```python
from build123d import *

# Parameters (mm, degrees)
F2_W     = 60.64
F2_H     = 2.8
F2_W_2   = 2.8
F2_H_2   = 60.64
F2_W_3   = 7.58
F2_H_3   = 7.58
F3_DEPTH = 2.8
F4_DEPTH = 6
F5_DEPTH = 35.6
F7_W     = 60.64
F7_H     = 2.8
F7_W_2   = 2.8
F7_H_2   = 60.64
F7_H_3   = 7.58
F7_W_3   = 7.58
F8_DEPTH = 2.8
F9_DEPTH = 6


with BuildPart() as f3:
    # F2 (on Top) → F3 (new body)
    with BuildSketch(Plane.XY):
        with Locations((0, 39.3)):
            Rectangle(F2_W, F2_H)
        Polygon((-40.7, 30.32), (-37.9, 30.32), (-37.9, 37.9), (-30.32, 37.9), (-30.32, 40.7), (-40.7, 40.7), align=None)
        Polygon((37.9, 37.9), (37.9, 30.32), (40.7, 30.32), (40.7, 40.7), (30.32, 40.7), (30.32, 37.9), align=None)
        with Locations((39.3, 0)):
            Rectangle(F2_W_2, F2_H_2)
        Polygon((37.9, -30.32), (37.9, -37.9), (30.32, -37.9), (30.32, -40.7), (40.7, -40.7), (40.7, -30.32), align=None)
        with Locations((0, -39.3)):
            Rectangle(F2_W, F2_H)
        Polygon((-30.32, -40.7), (-30.32, -37.9), (-37.9, -37.9), (-37.9, -30.32), (-40.7, -30.32), (-40.7, -40.7), align=None)
        with Locations((-39.3, 0)):
            Rectangle(F2_W_2, F2_H_2)
        with Locations((34.11, -34.11)):
            Rectangle(F2_W_3, F2_H_3)
        with Locations((34.11, 34.11)):
            Rectangle(F2_W_3, F2_H_3)
        with Locations((-34.11, 34.11)):
            Rectangle(F2_W_3, F2_H_3)
        with Locations((-34.11, 0)):
            Rectangle(F2_W_3, F2_H_2)
        with Locations((34.11, 0)):
            Rectangle(F2_W_3, F2_H_2)
        with Locations((-34.11, -34.11)):
            Rectangle(F2_W_3, F2_H_3)
        with Locations((0, -34.11)):
            Rectangle(F2_W, F2_H_3)
        with Locations((0, 34.11)):
            Rectangle(F2_W, F2_H_3)
    extrude(amount=F3_DEPTH)

    # F2 (on Top) → F4 (join)
    with BuildSketch(Plane.XY):
        with Locations((0, 39.3)):
            Rectangle(F2_W, F2_H)
        Polygon((-40.7, 30.32), (-37.9, 30.32), (-37.9, 37.9), (-30.32, 37.9), (-30.32, 40.7), (-40.7, 40.7), align=None)
        with Locations((-39.3, 0)):
            Rectangle(F2_W_2, F2_H_2)
        Polygon((-30.32, -40.7), (-30.32, -37.9), (-37.9, -37.9), (-37.9, -30.32), (-40.7, -30.32), (-40.7, -40.7), align=None)
        with Locations((0, -39.3)):
            Rectangle(F2_W, F2_H)
        Polygon((37.9, -30.32), (37.9, -37.9), (30.32, -37.9), (30.32, -40.7), (40.7, -40.7), (40.7, -30.32), align=None)
        with Locations((39.3, 0)):
            Rectangle(F2_W_2, F2_H_2)
        Polygon((37.9, 37.9), (37.9, 30.32), (40.7, 30.32), (40.7, 40.7), (30.32, 40.7), (30.32, 37.9), align=None)
    extrude(amount=F4_DEPTH)

    # F2 (on Top) → F5 (join)
    with BuildSketch(Plane.XY):
        Polygon((-40.7, 30.32), (-37.9, 30.32), (-37.9, 37.9), (-30.32, 37.9), (-30.32, 40.7), (-40.7, 40.7), align=None)
        Polygon((37.9, 37.9), (37.9, 30.32), (40.7, 30.32), (40.7, 40.7), (30.32, 40.7), (30.32, 37.9), align=None)
        Polygon((37.9, -30.32), (37.9, -37.9), (30.32, -37.9), (30.32, -40.7), (40.7, -40.7), (40.7, -30.32), align=None)
        Polygon((-30.32, -40.7), (-30.32, -37.9), (-37.9, -37.9), (-37.9, -30.32), (-40.7, -30.32), (-40.7, -40.7), align=None)
    extrude(amount=F5_DEPTH)

    # F7 (on offset) → F8 (join)
    with BuildSketch(Plane.XY.offset(35.6)):
        Polygon((37.9, -30.32), (37.9, -37.9), (30.32, -37.9), (30.32, -40.7), (40.7, -40.7), (40.7, -30.32), align=None)
        with Locations((0, -39.3)):
            Rectangle(F7_W, F7_H)
        with Locations((39.3, 0)):
            Rectangle(F7_W_2, F7_H_2)
        Polygon((-30.32, -40.7), (-30.32, -37.9), (-37.9, -37.9), (-37.9, -30.32), (-40.7, -30.32), (-40.7, -40.7), align=None)
        Polygon((37.9, 37.9), (37.9, 30.32), (40.7, 30.32), (40.7, 40.7), (30.32, 40.7), (30.32, 37.9), align=None)
        with Locations((-39.3, 0)):
            Rectangle(F7_W_2, F7_H_2)
        with Locations((0, 39.3)):
            Rectangle(F7_W, F7_H)
        Polygon((-40.7, 30.32), (-37.9, 30.32), (-37.9, 37.9), (-30.32, 37.9), (-30.32, 40.7), (-40.7, 40.7), align=None)
        with Locations((0, 34.11)):
            Rectangle(F7_W, F7_H_3)
        with Locations((34.11, 34.11)):
            Rectangle(F7_W_3, F7_H_3)
        with Locations((34.11, 0)):
            Rectangle(F7_W_3, F7_H_2)
        with Locations((34.11, -34.11)):
            Rectangle(F7_W_3, F7_H_3)
        with Locations((0, -34.11)):
            Rectangle(F7_W, F7_H_3)
        with Locations((-34.11, -34.11)):
            Rectangle(F7_W_3, F7_H_3)
        with Locations((-34.11, 0)):
            Rectangle(F7_W_3, F7_H_2)
        with Locations((-34.11, 34.11)):
            Rectangle(F7_W_3, F7_H_3)
    extrude(amount=-F8_DEPTH)

    # F7 (on offset) → F9 (join)
    with BuildSketch(Plane.XY.offset(35.6)):
        Polygon((-30.32, -40.7), (-30.32, -37.9), (-37.9, -37.9), (-37.9, -30.32), (-40.7, -30.32), (-40.7, -40.7), align=None)
        with Locations((-39.3, 0)):
            Rectangle(F7_W_2, F7_H_2)
        with Locations((0, -39.3)):
            Rectangle(F7_W, F7_H)
        with Locations((39.3, 0)):
            Rectangle(F7_W_2, F7_H_2)
        with Locations((0, 39.3)):
            Rectangle(F7_W, F7_H)
    extrude(amount=-F9_DEPTH)


solid = f3.part
```
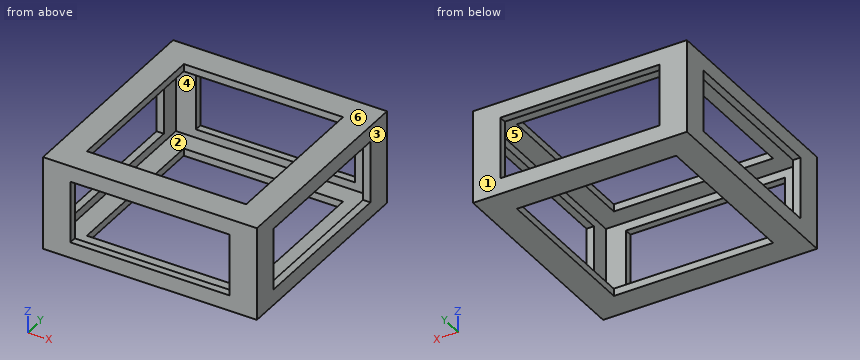
Geometry check sheet. Reference: the model listing, model coordinates, mm. Face numbers are marked on the shaded views. A direction names the side the tool comes from. Coordinates: 2 decimals unless noted, no trailing zeros. Write each loop counter-clockwise with the first axis right and the second up, starting at its lowest first coordinate (ties: lowest second). Pieces come first, ordered by that corner, then holes. Notation, with made-up numbers: M 45,-33.5 L 68,-33.5 A7 ccw 68,-22.5 Z; hole C 38,62.25 d5. An arc over 180 degrees is marked long. One line per item, written item: value. Start each with the question number.
(1) Sectioned sample at B-B, the plane x = -7. Enter the section's corners in (y, z), and give its area (3 significant figures).
(2) Release check for a two-part mould opening along Z. For the marked faces 3, 4, 5 and 6 record: released by +Z, released by -Z, zero draft, split by the parting line, or undercut.
(3) Sectioned sample at A-A, the plane z = 15.5. Enter the section's corners in (x, y).
(4) Sectioned sample at C-C, the plane y = -34.5. Enter the section's corners in (x, z).
(5) Scan lines: line 1 along Y through (x, z) = (16, 3.5); line 2 along Z through (x, y) = (36.5, -21). Record each from-to range of solid material in increasing order. Write a range as [from, to].
(6) Tool access check on the marked faces 1 and 2. Record the directions out of +Z, -Z, +X, -X, +Y, -Y that give a thin tool (end or side, any length) a straight path to the whole face; none if there is none.
Filled sheet:
1. outline: M -40.7,0 L -30.32,0 L -30.32,2.8 L -37.9,2.8 L -37.9,6 L -40.7,6 Z; M -40.7,29.6 L -37.9,29.6 L -37.9,32.8 L -30.32,32.8 L -30.32,35.6 L -40.7,35.6 Z; M 30.32,0 L 40.7,0 L 40.7,6 L 37.9,6 L 37.9,2.8 L 30.32,2.8 Z; M 30.32,32.8 L 37.9,32.8 L 37.9,29.6 L 40.7,29.6 L 40.7,35.6 L 30.32,35.6 Z
1. area: 152 mm²
2. face 3: zero draft
2. face 4: undercut
2. face 5: undercut
2. face 6: released by +Z
3. outline: M -40.7,-40.7 L -30.32,-40.7 L -30.32,-37.9 L -37.9,-37.9 L -37.9,-30.32 L -40.7,-30.32 Z; M -40.7,30.32 L -37.9,30.32 L -37.9,37.9 L -30.32,37.9 L -30.32,40.7 L -40.7,40.7 Z; M 30.32,-40.7 L 40.7,-40.7 L 40.7,-30.32 L 37.9,-30.32 L 37.9,-37.9 L 30.32,-37.9 Z; M 30.32,37.9 L 37.9,37.9 L 37.9,30.32 L 40.7,30.32 L 40.7,40.7 L 30.32,40.7 Z
4. outline: M -40.7,0 L 40.7,0 L 40.7,35.6 L -40.7,35.6 Z; hole M -37.9,2.8 L 37.9,2.8 L 37.9,32.8 L -37.9,32.8 Z
5. line 1: [-40.7, -37.9], [37.9, 40.7]
5. line 2: [0, 2.8], [32.8, 35.6]
6. face 1: +Z, -Z, +X, -X, +Y
6. face 2: none
